```python
from build123d import *

# Parameters (mm, degrees)
SKETCH1_R               = 15
SKETCH1_R_2             = 10
BOSS_EXTRUDE1_DEPTH     = 20
BOSS_EXTRUDE2_DEPTH     = 80
CUT_EXTRUDE1_DEPTH      = 226.610283454
CUT_EXTRUDE1_DEPTH_BACK = 226.610283454
SKETCH2_R               = 10


with BuildPart() as part:
    # Sketch1 → Boss-Extrude1 (new, symmetric)
    # profile 1 of 2: a face of its own
    with BuildSketch(Plane.YZ):
        with BuildLine():
            ThreePointArc((15, 0), (0, -15), (-15, 0))
            Line((-15, 0), (-15, -120))
            Line((-15, -120), (-55, -120))
            Line((-55, -120), (-55, -150))
            Line((-55, -150), (-5, -150))
            Line((-5, -150), (-5, -40))
            Line((-5, -40), (5, -40))
            Line((5, -40), (5, -150))
            Line((5, -150), (55, -150))
            Line((55, -150), (55, -120))
            Line((55, -120), (15, -120))
            Line((15, -120), (15, 0))
        make_face()
    # profile 2 of 2: a face of its own
    with BuildSketch(Plane.YZ):
        Circle(SKETCH1_R)
        with Locations(Location((0, 0, 0), (0, 0, 270))):
            Circle(SKETCH1_R_2, mode=Mode.SUBTRACT)
    extrude(amount=BOSS_EXTRUDE1_DEPTH, both=True)

    # Sketch1_3 → Boss-Extrude2 (add, symmetric)
    with BuildSketch(Plane.YZ):
        Polygon((55, -150), (5, -150), (5, -160), (35, -160), (35, -170), (15, -170), (15, -180), (55, -180), align=None)
        Polygon((-35, -160), (-5, -160), (-5, -150), (-55, -150), (-55, -180), (-15, -180), (-15, -170), (-35, -170), align=None)
    extrude(amount=BOSS_EXTRUDE2_DEPTH, both=True)

    # Sketch2 → Cut-Extrude1 (cut, two sides: drawn at the far end of the back side and taken through both)
    with BuildSketch(Plane(origin=(0, 55, 0), x_dir=(-1, 0, 0), z_dir=(0, 1, 0)).offset(-CUT_EXTRUDE1_DEPTH_BACK)):
        with Locations(Location((0, -135, 0), (0, 0, 90))):
            Circle(SKETCH2_R)
    extrude(amount=CUT_EXTRUDE1_DEPTH + CUT_EXTRUDE1_DEPTH_BACK, mode=Mode.SUBTRACT)


solid = part.part
```
Can you work these out from the model? Positions are in its coordinate system, mm. A direction names the side the tool comes from. Coordinates: 2 decimals unless noted, no trailing zeros. Order: outer loops, then holes, each group sorted by start corner. A loop starts at its lowest first (then second) coordinate and runs counter-clockwise, first axis right, second up.
1. If we section it at D-D (z = -49): Please give me the cut outline in (x, y), then the cut area to 3 significant figures.
2. For faces 1 (the face through (20, 11, -85)), 2 (the face through (-1, 20, -160)), 3 (the face through (1, -5, -114)), 4 (the face through (-50, -30, -150)), which set-ups out of +Z, -Z, +X, -X, +Y, -Y let a thin tool reach every point of the face, with its end or its side?
3. Thinking about a two-plate mould opening in Y: for faces 5 (the face through (1, 55, -157)), 6 (the face through (1, -15, -175)), 7 (the face through (80, 35.2, -164.8)), which applies, +Y half, -Y half, draft (parallel to the pull), parting line (faces both ways), or undercut?
4. If we section it at A-A (x = 52.5): Please give me the cut outline in (y, z), then the cut area to 3 significant figures.
5. I'm going to push flat-ended pins straight in: pin 1 (25 mm diameter, centred on x = -55, y = -19.5, fed in from +Z); pin 2 (8 mm diameter, centred on x = -17.5, z = -86, fed in from +Y); pin 3 (3 mm diameter, centred on x = 16.5, y = -21, fed in from +Z). Where does each tip first touch, or does it pass through?
6. I need wall thicknesses on line 1 (X direction, y = -31, z = -135); line 2 (Y direction, x = 52.5, z = -160.5); line 3 (Y direction, x = -9.75, z = 0). Which ranges of each line are inside material? Lowest first, please.
7. If we section it at C-C (y = 0): Please give me the cut outline in (x, z).
8. If we section it at B-B (y = 27): Please give me the cut outline in (x, z).
Entries:
1. outline: (-20, -15) - (20, -15) - (20, -5) - (-20, -5) - close; (-20, 5) - (20, 5) - (20, 15) - (-20, 15) - close
1. area: 800 mm2
2. face 1: +Z, +X, +Y, -Y
2. face 2: +X, -X
2. face 3: -Z, +X, -X
2. face 4: +Z, -X, +Y, -Y
3. face 5: +Y half
3. face 6: undercut
3. face 7: draft
4. outline: (-55, -180) - (-15, -180) - (-15, -170) - (-35, -170) - (-35, -160) - (-5, -160) - (-5, -150) - (-55, -150) - close; (5, -160) - (35, -160) - (35, -170) - (15, -170) - (15, -180) - (55, -180) - (55, -150) - (5, -150) - close
4. area: 2,200 mm2
5. pin 1: stops at z = -150
5. pin 2: stops at y = 15
5. pin 3: stops at z = -120
6. line 1: x = -20 to -10, 10 to 20
6. line 2: y = -55 to -35, 35 to 55
6. line 3: y = -15 to -10, 10 to 15
7. outline: (-20, -40) - (20, -40) - (20, -10) - (-20, -10) - close; (-20, 10) - (20, 10) - (20, 15) - (-20, 15) - close
8. outline: (-80, -180) - (80, -180) - (80, -170) - (-80, -170) - close; (-80, -160) - (80, -160) - (80, -150) - (20, -150) - (20, -120) - (-20, -120) - (-20, -150) - (-80, -150) - close; hole circle Ø20 at (0, -135)
